```python
from build123d import *

# Parameters (mm, degrees)
SWEEP_THIN1_PROFILE_R   = 4
SWEEP_THIN1_PROFILE_R_2 = 3.5


with BuildPart() as part:
    # Sweep-Thin1: sweep along a path in Sketch1
    with BuildLine(Plane(origin=(0, 0, 0), x_dir=(1, 0, 0), z_dir=(0, 1, 0))) as sweep_thin1_path:
        Line((0, 0), (15, 0))
        ThreePointArc((15, 0), (18.535533906, 1.464466094), (20, 5))
        Line((20, 5), (20, 20))
    # Sweep-Thin1 profile (on start of the path) → Sweep-Thin1 (sweep)
    with BuildSketch(Plane(origin=(0, 0, 0), x_dir=(0, 0, 1), z_dir=(1, 0, 0))):
        Circle(SWEEP_THIN1_PROFILE_R)
        Circle(SWEEP_THIN1_PROFILE_R_2, mode=Mode.SUBTRACT)
    sweep(path=sweep_thin1_path.line)


solid = part.part
```
The model under review builds one solid part; all positions refer to its coordinate system, in mm. A direction names the side the tool comes from. Coordinates: 2 decimals unless noted, no trailing zeros. Loops run counter-clockwise (first coordinate to the right, second up) from the corner with the lowest first, then second, coordinate; pieces in that order, holes last. Notation, with made-up numbers: (3, -20.75) -> (55, -20.75) arc R29 ccw to (55, 4.25) -> close; hole circle Ø9 at (72.25, 59.5). An arc over 180 degrees is marked (long way). Answer as CSV lines item,"result".
Item 1: Take a section at B-B, the plane x = 8. State the section outline as (y, z) points, and give its area (3 significant figures).
Results below:
outline,"circle Ø8 at (0, 0); hole circle Ø7 at (0, 0)"
area,"11.8 mm2"
Item 2: Draft analysis for pull direction Y (two halves, no side actions). For faces 1 (the cylindrical face through (23.34, -1.05, -12.6)), 2 (the cylindrical face through (7.605, 3.905, -0.867)), state which applies: +Y half, -Y half, draft (parallel to the pull), parting line (faces both ways), or undercut.
Results below:
face 1,"undercut"
face 2,"parting line"
Item 3: Take a section at D-D, the plane y = 2.25. State the section outline as (x, z) points, and give its area (3 significant figures).
Results below:
outline,"(0, -3.31) -> (15, -3.31) arc R1.69 cw to (16.69, -5) -> (16.69, -20) -> (17.32, -20) -> (17.32, -5) arc R2.32 ccw to (15, -2.68) -> (0, -2.68) -> close; (0, 2.68) -> (15, 2.68) arc R7.68 cw to (22.68, -5) -> (22.68, -20) -> (23.31, -20) -> (23.31, -5) arc R8.31 ccw to (15, 3.31) -> (0, 3.31) -> close"
area,"47.4 mm2"
Item 4: Machinability: for faces 3 (the cylindrical face through (16.8, 2.4, -12.6)), 4 (the cylindrical face through (7.605, 1.341, 3.233)), which of the approach directions +Z, -Z, +X, -X, +Y, -Y give a long, thin tool a straight path to every point of the face, cutting with its end or side? Answer none if there is none.
Results below:
face 3,"-Z"
face 4,"-X"
Item 5: Take a section at C-C, the plane z = -17.5. State the section outline as (x, y) points.
Results below:
outline,"circle Ø8 at (20, 0); hole circle Ø7 at (20, 0)"
Item 6: For L1, parallel to Z at x = 4.5, y = 0; L2, parallel to X at y = 0, z = -18.5, list the stretches that pass through material, from the lowest coordinate up.
Results below:
L1,"z = -4 to -3.5, 3.5 to 4"
L2,"x = 16 to 16.5, 23.5 to 24"
Item 7: Take a section at A-A, the plane y = 0. State the section outline as (x, z) points, and give its area (3 significant figures).
Results below:
outline,"(0, -4) -> (15, -4) arc R1 cw to (16, -5) -> (16, -20) -> (16.5, -20) -> (16.5, -5) arc R1.5 ccw to (15, -3.5) -> (0, -3.5) -> close; (0, 3.5) -> (15, 3.5) arc R8.5 cw to (23.5, -5) -> (23.5, -20) -> (24, -20) -> (24, -5) arc R9 ccw to (15, 4) -> (0, 4) -> close"
area,"37.9 mm2"
Item 8: Insertion check: pin 1 (3 mm diameter, centred on x = 10.5, y = 2, fed in from -Z); pin 2 (1.5 mm diameter, centred on x = 17, z = -15, fed in from +Y); pin 3 (1.5 mm diameter, centred on y = 3, z = -14, fed in from +X). Each pin has a flat end and moves straight along its axis. Give the tip position at first contact, or say it passes through.
Results below:
pin 1,"stops at z = -3.97"
pin 2,"stops at y = 3.31"
pin 3,"stops at x = 23.31"
